Verification items for the finished model (mm, model axes). A direction names the side the tool comes from. Coordinates: 2 decimals unless noted, no trailing zeros. Order: outer loops, then holes, each group sorted by start corner. A loop starts at its lowest first (then second) coordinate and runs counter-clockwise, first axis right, second up. Notation, with made-up numbers: M -27,53 L 32,53 A16 cw 32,68 Z; hole C -12.5,47 d5. An arc over 180 degrees is marked long. Write item = value, one per line.
```python
from build123d import *


with BuildPart() as part:
    # Sketch1 → Revolve1 (revolve)
    with BuildSketch(Plane.XY):
        with BuildLine():
            Line((30, 76), (30, 0))
            Line((30, 0), (55, 0))
            Line((55, 0), (55, 45))
            ThreePointArc((55, 45), (58.132644659, 50.270509781), (64.259424449, 50.03747479))
            Line((64.259424449, 50.03747479), (87.5, 35))
            Line((87.5, 35), (87.5, -12))
            Line((87.5, -12), (92.5, -12))
            Line((92.5, -12), (92.5, 27.206415499))
            Line((92.5, 27.206415499), (103, 27.206415499))
            Line((103, 27.206415499), (103, 62.206415499))
            Line((103, 62.206415499), (92.5, 62.206415499))
            ThreePointArc((92.5, 62.206415499), (90.409938476, 58.140427542), (85.887096774, 57.473705579))
            Line((85.887096774, 57.473705579), (55, 68))
            Line((55, 68), (55, 76))
            Line((55, 76), (30, 76))
        make_face()
    revolve(axis=Axis((0, -19.792449206, 0), (0, 1, 0)))


solid = part.part
```
Item 1: Scan lines: L1, parallel to X at y = 25, z = 0; L2, parallel to X at y = 55, z = 0. Record each from-to range of solid material in increasing order. Write a range as from..to.
Report:
L1 = -92.5..-87.5, -55..-30, 30..55, 87.5..92.5
L2 = -103..-30, 30..103
Item 2: Tool access check on faces 4 (the cylindrical face through (49.727, 7.878, -77.996)), 5 (the cylindrical face through (-11.923, 72.056, 53.692)), 6 (the cylindrical face through (-29.97, 37.47, -1.32)). Record the directions out of +Z, -Z, +X, -X, +Y, -Y that give a thin tool (end or side, any length) a straight path to the whole face; none if there is none.
Report:
face_4 = -Y
face_5 = +Y
face_6 = +Y, -Y
Item 3: Sectioned sample at D-D, the plane y = 15.5. Enter the section's corners in (x, z), then the cut area to 3 significant figures.
Report:
outline = C 0,0 d185; C 0,0 d110; hole C 0,0 d175; hole C 0,0 d60
area = 9,500 mm^2
Item 4: Gauge pin test, flat ends, axial feed: pin 1 (6 mm diameter, centred on y = 32, z = 32.5, fed in from -X); pin 2 (3 mm diameter, centred on x = 22, z = 15, fed in from -Y); pin 3 (1.5 mm diameter, centred on x = -49, z = 31.5, fed in from +Y); pin 4 (4 mm diameter, centred on y = 48, z = -48, fed in from +X). Record the tip position at first contact, or that the pin passes through.
Report:
pin_1 = -98.69
pin_2 = through
pin_3 = 67.15
pin_4 = 92.16
Item 5: Release check for a two-part mould opening along Z. For faces 1 (the flat face through (55.2, -12, 68.1)), 2 (the cylindrical face through (-22.33, 44.95, 100.55)), 3 (the cylindrical face through (-11.923, 22.815, 53.692)) record: pulls with the +Z half, pulls with the -Z half, needs draft (parallel to the pull), parting line crosses it, or undercut.
Report:
face_1 = needs draft
face_2 = parting line crosses it
face_3 = undercut
Item 6: Sectioned sample at B-B, the plane y = 31. Enter the section's corners in (x, z).
Report:
outline = C 0,0 d206; C 0,0 d110; hole C 0,0 d175; hole C 0,0 d60
